Can you work these out from the model? Positions are in its coordinate system, mm. A direction names the side the tool comes from. Give positions to 0.01 mm unless a question says otherwise; leave off trailing zeros. Order: outer loops, then holes, each group sorted by start corner. A loop starts at its lowest first (then second) coordinate and runs counter-clockwise, first axis right, second up. Notation, with made-up numbers: (70, 58.5) - (126, 58.5) arc R24 ccw to (126, 83.5) - close; hole circle Ø7 at (17, -36.5). An arc over 180 degrees is marked (long way). Answer as a JSON object with one key per item and string values.
```python
from build123d import *

# Parameters (mm, degrees)
CROQUIS1_W              = 32.1
CROQUIS1_H              = 12.3
SALIENTE_EXTRUIR1_DEPTH = 1
CROQUIS2_W              = 1.8
CROQUIS2_H              = 0.5
SALIENTE_EXTRUIR2_DEPTH = 1
SALIENTE_EXTRUIR3_DEPTH = 2
REDONDEO2_R             = 0.5
REDONDEO3_R             = 1
REDONDEO4_R             = 0.3
REDONDEO6_R             = 0.3


with BuildPart() as part:
    # Croquis1 → Saliente-Extruir1 (new body)
    with BuildSketch(Plane(origin=(0, 0, 0), x_dir=(1, 0, 0), z_dir=(0, 1, 0))):
        with Locations((0.329771615, 2.864192496)):
            Rectangle(CROQUIS1_W, CROQUIS1_H)
    extrude(amount=SALIENTE_EXTRUIR1_DEPTH)

    # Croquis2 → Saliente-Extruir2 (add)
    with BuildSketch(Plane(origin=(-6.706035889, 0, -9.014192496), x_dir=(1, 0, 0), z_dir=(0, 0, 1))):
        with Locations((-6.114192496, 0.25)):
            Rectangle(CROQUIS2_W, CROQUIS2_H)
        with Locations((20.185807504, 0.25)):
            Rectangle(CROQUIS2_W, CROQUIS2_H)
    extrude(amount=-SALIENTE_EXTRUIR2_DEPTH)

    # Croquis4 → Saliente-Extruir3 (add, symmetric)
    with BuildSketch(Plane.ZY.offset(-0.329771615)):
        Polygon((3.285807504, 1), (3.285807504, 0), (4.035807504, -1.718465886), (5.004025394, 0.5), (7.285807504, 0.5), (7.285807504, 1), (4.785807504, 1), (4.035807504, -0.718465886), align=None)
    extrude(amount=SALIENTE_EXTRUIR3_DEPTH, both=True)

    # Redondeo2
    redondeo2_edges = [part.edges().sort_by_distance(p)[0] for p in [
        (0.329771615, -1.718465886, 4.035807504),
    ]]
    fillet(redondeo2_edges, radius=REDONDEO2_R)

    # Redondeo3
    redondeo3_edges = [part.edges().sort_by_distance(p)[0] for p in [
        (2.329771615, 0.75, 7.285807504),
        (-1.670228385, 0.75, 7.285807504),
    ]]
    fillet(redondeo3_edges, radius=REDONDEO3_R)

    # Redondeo4
    redondeo4_edges = [part.edges().sort_by_distance(p)[0] for p in [
        (2.329771615, 0.5, 5.644916449),
        (-1.670228385, 0.5, 5.644916449),
        (0.329771615, 0.5, 7.285807504),
        (2.036878396, 0.5, 6.992914285),
        (-1.377335166, 0.5, 6.992914285),
    ]]
    fillet(redondeo4_edges, radius=REDONDEO4_R)

    # Redondeo6
    redondeo6_edges = [part.edges().sort_by_distance(p)[0] for p in [
        (-14.720228385, 0, -9.014192496),
        (-12.820228385, 0, -10.014192496),
        (0.329771615, 0, -9.014192496),
        (13.479771615, 0, -10.014192496),
        (9.354771615, 0, 3.285807504),
        (15.379771615, 0, -9.014192496),
        (16.379771615, 0, -2.864192496),
        (-8.695228385, 0, 3.285807504),
        (-15.720228385, 0, -2.864192496),
    ]]
    fillet(redondeo6_edges, radius=REDONDEO6_R)


solid = part.part
```
Q1. We'd pull the mould along Z, two halves only. Please class faces 1 (the face through (0.302, 0.153, 4.416)), 2 (the face through (-1.67, -0.1, 4.5)), 3 (the face through (0.302, 0.129, 3.666)), 4 (the face through (0.302, -0.108, 4.739)): released by +Z, released by -Z, zero draft, split by the parting line, or undercut.
Recorded:
{"face 1": "undercut", "face 2": "zero draft", "face 3": "undercut", "face 4": "released by +Z"}
Q2. I'm going to push flat-ended pins straight in: pin 1 Ø0.5 at (x, z) = (13.5, -9.5) entering from +Y; pin 2 Ø0.8 at (x, y) = (3, 1) entering from -Z; pin 3 Ø0.6 at (y, z) = (0.5, 4.5) entering from +X. Where does each tip first touch, or does it pass through?
Recorded:
{"pin 1": "stops at y = 0.5", "pin 2": "stops at z = -9.01", "pin 3": "stops at x = 2.33"}
Q3. If we section it at C-C, the plane x = -8: Please give me the cut outline in (y, z).
Recorded:
{"outline": "(0, -8.71) arc R0.3 ccw to (0.3, -9.01) - (1, -9.01) - (1, 3.29) - (0.3, 3.29) arc R0.3 ccw to (0, 2.99) - close"}
Q4. If we section it at A-A, the plane z = 2.5: Please give me the cut outline in (x, y), then the cut area to 3 significant figures.
Recorded:
{"outline": "(-15.72, 0.3) arc R0.3 ccw to (-15.42, 0) - (16.08, 0) arc R0.3 ccw to (16.38, 0.3) - (16.38, 1) - (-15.72, 1) - close", "area": "32.1 mm^2"}
Q5. If we section it at B-B, the plane y = -0.35: Please give me the cut outline in (x, z) (3 decimals).
Recorded:
{"outline": "(-1.67, 3.439) - (2.33, 3.439) - (2.33, 3.875) - (-1.67, 3.875) - close; (-1.67, 4.197) - (2.33, 4.197) - (2.33, 4.633) - (-1.67, 4.633) - close"}
Q6. I need wall thicknesses on L1, parallel to Z at x = 9.5, y = 0.55; L2, parallel to Y at x = -1.5, z = -6.75; L3, parallel to X at y = 0.25, z = 1.5. Which ranges of each line are inside material? Lowest first, please.
Recorded:
{"L1": "z = -9.01 to 3.29", "L2": "y = 0 to 1", "L3": "x = -15.72 to 16.38"}
Q7. Which directions (+Z, -Z, +X, -X, +Y, -Y) give clear straight access to the entire face, cutting with the end or side of a thin tool? Please do faces 5 (the face through (0, 0.5, 6)), 6 (the face through (0, 1, 6)), 7 (the face through (-12.8, 0.5, -9.5)).
Recorded:
{"face 5": "+Z, +X, -X, -Y", "face 6": "+Z, -Z, +X, -X, +Y", "face 7": "-Z, +X, -X, +Y"}
